```python
from build123d import *

# Parameters (mm, degrees)
F0_R     = 19.5
F0_R_2   = 15
F1_DEPTH = 9
F2_DEPTH = 83
F0_R_3   = 23.25
F3_DEPTH = 74
F0_R_4   = 5
F0_R_5   = 2.5
F4_DEPTH = 27
F5_DEPTH = 4
F6_DEPTH = 27


with BuildPart() as f1:
    # F0 (on Front) → F1 (new body)
    with BuildSketch(Plane.XZ):
        Circle(F0_R)
        Circle(F0_R_2, mode=Mode.SUBTRACT)
    extrude(amount=F1_DEPTH)

    # F0 (on Front) → F2 (join)
    with BuildSketch(Plane.XZ):
        Circle(F0_R)
        Circle(F0_R_2, mode=Mode.SUBTRACT)
    extrude(amount=-F2_DEPTH)

    # F0 (on Front) → F3 (join)
    with BuildSketch(Plane.XZ):
        Circle(F0_R_3)
        Circle(F0_R, mode=Mode.SUBTRACT)
    extrude(amount=-F3_DEPTH)

    # F0 (on Front) → F4 (join)
    with BuildSketch(Plane.XZ):
        with BuildLine():
            Line((27.5, -22.449944), (27.5, 22.449944))
            ThreePointArc((27.5, 22.449944), (-35.5, 0), (27.5, -22.449944))
        make_face()
        with Locations((15, -24.819347)):
            Circle(F0_R_4, mode=Mode.SUBTRACT)
        with Locations((-29, 0)):
            Circle(F0_R_4, mode=Mode.SUBTRACT)
        Circle(F0_R_3, mode=Mode.SUBTRACT)
        with Locations((15, 24.819347)):
            Circle(F0_R_4, mode=Mode.SUBTRACT)
        with Locations((15, 24.819347)):
            Circle(F0_R_4)
        with Locations((15, 24.819347)):
            Circle(F0_R_5, mode=Mode.SUBTRACT)
        with Locations((15, 24.819347)):
            Circle(F0_R_5)
        with Locations((15, -24.819347)):
            Circle(F0_R_4)
        with Locations((15, -24.819347)):
            Circle(F0_R_5, mode=Mode.SUBTRACT)
        with Locations((15, -24.819347)):
            Circle(F0_R_5)
        with Locations((-29, 0)):
            Circle(F0_R_4)
        with Locations((-29, 0)):
            Circle(F0_R_5, mode=Mode.SUBTRACT)
        with Locations((-29, 0)):
            Circle(F0_R_5)
    extrude(amount=-F4_DEPTH)

    # F0 (on Front) → F5 (cut)
    with BuildSketch(Plane.XZ):
        with Locations((15, -24.819347)):
            Circle(F0_R_4)
        with Locations((15, -24.819347)):
            Circle(F0_R_5, mode=Mode.SUBTRACT)
        with Locations((15, 24.819347)):
            Circle(F0_R_4)
        with Locations((15, 24.819347)):
            Circle(F0_R_5, mode=Mode.SUBTRACT)
        with Locations((-29, 0)):
            Circle(F0_R_4)
        with Locations((-29, 0)):
            Circle(F0_R_5, mode=Mode.SUBTRACT)
    extrude(amount=-F5_DEPTH, mode=Mode.SUBTRACT)

    # F0 (on Front) → F6 (cut)
    with BuildSketch(Plane.XZ):
        with Locations((15, -24.819347)):
            Circle(F0_R_5)
        with Locations((15, 24.819347)):
            Circle(F0_R_5)
        with Locations((-29, 0)):
            Circle(F0_R_5)
    extrude(amount=-F6_DEPTH, mode=Mode.SUBTRACT)


solid = f1.part
```
The listing builds one solid part. Answer for the finished solid, in the listing's coordinates (mm). A direction names the side the tool comes from. Give positions to 0.01 mm unless a question says otherwise; leave off trailing zeros. Order: outer loops, then holes, each group sorted by start corner. A loop starts at its lowest first (then second) coordinate and runs counter-clockwise, first axis right, second up. Notation, with made-up numbers: M 15,16 L 50,16 A14 ccw 50,27 Z; hole C 32.5,-31 d8. An arc over 180 degrees is marked long. Put each result on its own line as item: value. Start each with the question number.
Item 1: Find the intervals of material crossed by line 1 along Z through (x, y) = (0, 13); line 2 along X through (y, z) = (23.5, -1); line 3 along X through (y, z) = (64, 10.5), in increasing order.
Item 2: Flat-ended cylindrical pins translate along their axes: P1, Ø4, axis at y = 55.5, z = -21.5, coming from the +X side; P2, Ø8, axis at x = 7, z = -11.5, coming from the +Y side; P3, Ø1, axis at x = -0.5, y = 39.5, coming from the -Z side; P4, Ø9, axis at x = 15, z = -24.82, coming from the +Y side. Find the tip coordinate at first contact, or state that the pin passes through.
Item 3: The part is cut by section B-B, the plane x = 0. Determine the outline of the cut face in (y, z), and give its area (3 significant figures).
Item 4: Which of the six approach directions +Z, -Z, +X, -X, +Y, -Y give full straight-line access (tool end or side, diameter ignored) to faces 1 (the face through (-2.539, 78.437, 19.334)), 2 (the face through (10, 83, -11.5)), 3 (the face through (17.688, 1.972, 29.035))?
Item 5: The part is cut by section C-C, the plane z = 12.5. Determine the outline of the cut face in (x, y), and give its area (3 significant figures).
Item 6: The part is cut by section D-D, the plane y = 1.5. Determine the outline of the cut face in (x, z).
Item 7: The part is cut by section A-A, the plane z = 0. Determine the outline of the cut face in (x, y).
Item 8: For a pull along Z with two mould halves and no side action, classify faces 4 (the face through (-2.539, -4.563, 19.334)), 5 (the face through (27.5, 13, 0)), 6 (the face through (12.502, 15.339, -24.709)) as +Z half, -Z half, draft (parallel to the pull), parting line (faces both ways), or undercut.
Answer key:
1. line 1: z = -35.5 to -15, 15 to 35.5
1. line 2: x = -35.49 to -31.29, -26.71 to -14.97, 14.97 to 27.5
1. line 3: x = -20.74 to -10.71, 10.71 to 20.74
2. P1: stops at x = 12.66
2. P2: stops at y = 83
2. P3: stops at z = -23.25
2. P4: stops at y = 27
3. outline: M -9,-19.5 L 0,-19.5 L 0,-35.5 L 27,-35.5 L 27,-23.25 L 74,-23.25 L 74,-19.5 L 83,-19.5 L 83,-15 L -9,-15 Z; M -9,15 L 83,15 L 83,19.5 L 74,19.5 L 74,23.25 L 27,23.25 L 27,35.5 L 0,35.5 L 0,19.5 L -9,19.5 Z
3. area: 2,040 mm²
4. face 1: +Y
4. face 2: +Z, -Z, +X, -X, +Y
4. face 3: -Y
5. outline: M -33.23,0 L -14.97,0 L -14.97,-9 L -8.29,-9 L -8.29,83 L -14.97,83 L -14.97,74 L -19.6,74 L -19.6,27 L -33.23,27 Z; M 8.29,-9 L 14.97,-9 L 14.97,0 L 27.5,0 L 27.5,27 L 19.6,27 L 19.6,74 L 14.97,74 L 14.97,83 L 8.29,83 Z
5. area: 2,500 mm²
6. outline: M 27.5,-22.45 L 27.5,22.45 A35.5 ccw long Z; hole C -29,0 d10; hole C 0,0 d30; hole C 15,-24.82 d10; hole C 15,24.82 d10
7. outline: M -35.5,0 L -34,0 L -34,4 L -31.5,4 L -31.5,27 L -35.5,27 Z; M -26.5,4 L -24,4 L -24,0 L -19.5,0 L -19.5,-9 L -15,-9 L -15,83 L -19.5,83 L -19.5,74 L -23.25,74 L -23.25,27 L -26.5,27 Z; M 15,-9 L 19.5,-9 L 19.5,0 L 27.5,0 L 27.5,27 L 23.25,27 L 23.25,74 L 19.5,74 L 19.5,83 L 15,83 Z
8. face 4: parting line
8. face 5: draft
8. face 6: undercut
